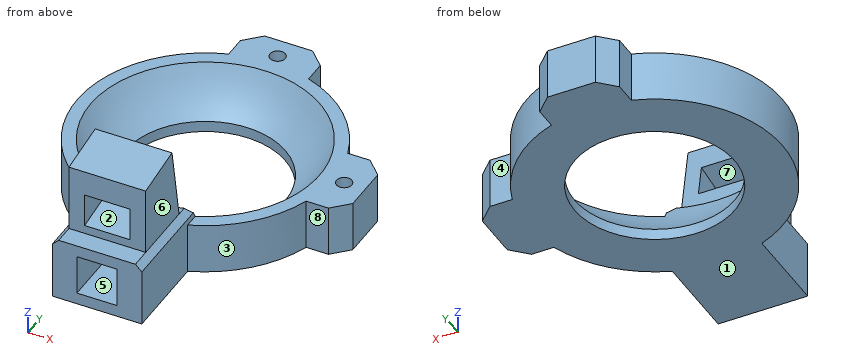
from build123d import *

# Parameters (mm, degrees)
SKETCH1_R            = 12.5
BOSS_EXTRUDE1_DEPTH  = 8
BOSS_EXTRUDE2_DEPTH  = 10
SKETCH4_W            = 6.3
SKETCH4_H            = 6.3
CUT_EXTRUDE1_DEPTH   = 12
BOSS_EXTRUDE4_DEPTH  = 6
SKETCH13_W           = 7.1
SKETCH13_H           = 5.2
CUT_EXTRUDE5_DEPTH   = 51.192153127
SKETCH22_W           = 12.489995996
SKETCH22_H           = 4
BOSS_EXTRUDE10_DEPTH = 8
SKETCH24_R           = 1.2
CUT_EXTRUDE8_DEPTH   = 6.5
CIRPATTERN1_COUNT    = 2
CIRPATTERN1_ANGLE    = 90
CHAMFER1_SIZE        = 2.5
CHAMFER2_SIZE        = 1


with BuildPart() as part:
    # Sketch1 → Boss-Extrude1 (new body)
    with BuildSketch(Plane.XY):
        with BuildLine():
            Line((-6.244997998, 21), (6.244997998, 21))
            Line((6.244997998, 21), (6.244997998, 19))
            ThreePointArc((6.244997998, 19), (14.142135624, 14.142135624), (19, 6.244997998))
            Line((19, 6.244997998), (21, 6.244997998))
            Line((21, 6.244997998), (21, -6.244997998))
            Line((21, -6.244997998), (19, -6.244997998))
            ThreePointArc((19, -6.244997998), (11.728172066, -16.200308021), (0, -20))
            ThreePointArc((0, -20), (-19.748417658, -3.16227766), (-6.244997998, 19))
            Line((-6.244997998, 19), (-6.244997998, 21))
        make_face()
        Circle(SKETCH1_R, mode=Mode.SUBTRACT)
    extrude(amount=BOSS_EXTRUDE1_DEPTH)

    # Sketch3 → Boss-Extrude2 (add)
    with BuildSketch(Plane.XY):
        Polygon((-7, -18.734993995), (-7, -32.5), (7, -32.5), (7, -18.734993995), (7, -15.234993995), (-7, -15.234993995), align=None)
    extrude(amount=BOSS_EXTRUDE2_DEPTH)

    # Sketch2 → Cut-Revolve2 (revolve, cut)
    with BuildSketch(Plane(origin=(0, 0, 0), x_dir=(1, 0, 0), z_dir=(0, 1, 0))):
        with BuildLine():
            Line((0, -38.5), (0, 2.5))
            ThreePointArc((0, 2.5), (-20.5, -18), (0, -38.5))
        make_face()
    revolve(axis=Axis((0, 0, 8), (0, 0, -1)), mode=Mode.SUBTRACT)

    # Sketch4 → Cut-Extrude1 (cut)
    with BuildSketch(Plane.XZ.offset(32.5)):
        with Locations((0, 5)):
            Rectangle(SKETCH4_W, SKETCH4_H)
    extrude(amount=-CUT_EXTRUDE1_DEPTH, mode=Mode.SUBTRACT)

    # Sketch11 → Boss-Extrude4 (add, symmetric)
    with BuildSketch(Plane(origin=(0, 0, 0), x_dir=(0, 0, -1), z_dir=(1, 0, 0))):
        Polygon((-10, -19.405629698), (-22, -21.521553466), (-20.609824642, -29.405629698), (-10, -29.405629698), align=None)
    extrude(amount=BOSS_EXTRUDE4_DEPTH, both=True)

    # Sketch13 → Cut-Extrude5 (cut, through all)
    with BuildSketch(Plane(origin=(0, -17.110377647, -3.017021229), x_dir=(1, 0, 0), z_dir=(0, 0.9848077530122074, 0.17364817766693455))):
        with Locations((0, -18.884652651)):
            Rectangle(SKETCH13_W, SKETCH13_H)
    extrude(amount=-CUT_EXTRUDE5_DEPTH, mode=Mode.SUBTRACT)

    # Sketch22 → Boss-Extrude10 (add)
    with BuildSketch(Plane.XY):
        with Locations((0, 23)):
            Rectangle(SKETCH22_W, SKETCH22_H)
    boss_extrude10 = extrude(amount=BOSS_EXTRUDE10_DEPTH)

    # Sketch24 → Cut-Extrude8 (cut)
    with BuildSketch(Plane.XY.offset(8)):
        with Locations((0, 21.7)):
            Circle(SKETCH24_R)
    cut_extrude8 = extrude(amount=-CUT_EXTRUDE8_DEPTH, mode=Mode.SUBTRACT)

    # CirPattern1: Boss-Extrude10, Cut-Extrude8 ×2 about axis
    cirpattern1_axis = Axis((0, 0, 0), (0, 0, -1))
    add([boss_extrude10.rotate(cirpattern1_axis, i * CIRPATTERN1_ANGLE / (CIRPATTERN1_COUNT - 1)) for i in range(1, CIRPATTERN1_COUNT)])
    add([cut_extrude8.rotate(cirpattern1_axis, i * CIRPATTERN1_ANGLE / (CIRPATTERN1_COUNT - 1)) for i in range(1, CIRPATTERN1_COUNT)], mode=Mode.SUBTRACT)

    # Chamfer1
    chamfer1_edges = [part.edges().sort_by_distance(p)[0] for p in [
        (-6.244997998, 25, 4),
        (6.244997998, 25, 4),
        (25, 6.244997998, 4),
        (25, -6.244997998, 4),
    ]]
    chamfer(chamfer1_edges, length=CHAMFER1_SIZE)

    # Chamfer2
    chamfer2_edges = [part.edges().sort_by_distance(p)[0] for p in [
        (7, -25.014274071, 10),
        (-7, -25.014274071, 10),
    ]]
    chamfer(chamfer2_edges, length=CHAMFER2_SIZE - 0.0001)  # a hair under: the kernel refuses the full size


solid = part.part
The model under review builds one solid part; all positions refer to its coordinate system, in mm. Face numbers are marked on the shaded views. A direction names the side the tool comes from. Give positions to 0.01 mm unless a question says otherwise; leave off trailing zeros. Loops run counter-clockwise (first coordinate to the right, second up) from the corner with the lowest first, then second, coordinate; pieces in that order, holes last. Notation, with made-up numbers: (0, 80) -> (24, 80) arc R16 ccw to (24, 101) -> close; hole circle Ø3 at (-19, 12). An arc over 180 degrees is marked (long way). Put each result on its own line as item: value. Start each with the question number.
1. Mouldability with a two-part tool opening along Z and no side actions: class the marked faces 1, 2 and 3 as released by +Z, released by -Z, zero draft, split by the parting line, or undercut.
2. We need section C-C on x = 0. State the section outline as (y, z) points.
3. We need section A-A on y = 0. State the section outline as (x, z) points, then the cut area to 3 significant figures.
4. We need section D-D on y = 21.7. State the section outline as (x, z) points (3 decimals), then the cut area to 3 significant figures.
5. Clearance check with flat-ended pins moving along their axes: P1, Ø1.9, axis at x = 21, y = -0.5, coming from the +Z side; P2, Ø2.5, axis at y = -26, z = 5, coming from the +X side; P3, Ø10, axis at x = 13.5, z = 19, coming from the +Y side; P4, Ø2, axis at y = -26, z = 14.5, coming from the -X side. State where each tip first meets the part, or that it passes through.
6. For the marked faces 4, 5, 6, 7 and 8, list the 3-axis set-ups (+Z, -Z, +X, -X, +Y, -Y) from which the entire face can be reached by the end or side of a thin tool; tool diameter is ignored.
7. We need section B-B on z = 15.25. State the section outline as (x, y) points.
8. Wall thickness on probe 1 along Y at (x, z) = (0, 6.25); probe 2 along X at (y, z) = (-25, 16.25); probe 3 along X at (y, z) = (-21.5, 6.75): over which ranges is each line inside the solid? List them lowest first.
Determined:
1. face 1: released by -Z
1. face 2: undercut
1. face 3: zero draft
2. outline: (-32.5, 0) -> (-12.5, 0) -> (-12.5, 1.75) arc R20.5 cw to (-18.87, 10) -> (-19.41, 10) -> (-19.94, 13.02) -> (-29.41, 11.35) -> (-29.41, 10) -> (-32.5, 10) -> (-32.5, 8.15) -> (-20.5, 8.15) -> (-20.5, 1.85) -> (-32.5, 1.85) -> close; (-29.41, 16.63) -> (-20.84, 18.14) -> (-21.52, 22) -> (-29.41, 20.61) -> close; (12.5, 0) -> (25, 0) -> (25, 8) -> (22.9, 8) -> (22.9, 1.5) -> (20.5, 1.5) -> (20.5, 8) -> (17.9, 8) arc R20.5 cw to (12.5, 1.75) -> close
3. outline: (-20, 0) -> (-12.5, 0) -> (-12.5, 1.75) arc R20.5 cw to (-17.9, 8) -> (-20, 8) -> close; (12.5, 0) -> (25, 0) -> (25, 8) -> (22.9, 8) -> (22.9, 1.5) -> (20.5, 1.5) -> (20.5, 8) -> (17.9, 8) arc R20.5 cw to (12.5, 1.75) -> close
3. area: 106 mm^2
4. outline: (-6.245, 0) -> (6.245, 0) -> (6.245, 8) -> (1.2, 8) -> (1.2, 1.5) -> (-1.2, 1.5) -> (-1.2, 8) -> (-6.245, 8) -> close
4. area: 84.3 mm^2
5. P1: z = 8
5. P2: x = 7
5. P3: through
5. P4: x = -6
6. face 4: +Z, -Z, +X, +Y
6. face 5: -Y
6. face 6: +Z, +X, +Y, -Y
6. face 7: +Y
6. face 8: +Z, -Z, +X, -Y
7. outline: (-6, -29.41) -> (-3.55, -29.41) -> (-3.55, -20.33) -> (-6, -20.33) -> close; (3.55, -29.41) -> (6, -29.41) -> (6, -20.33) -> (3.55, -20.33) -> close
8. probe 1: -20.5 to -16.8, 16.8 to 20.5, 22.9 to 25
8. probe 2: -6 to -3.55, 3.55 to 6
8. probe 3: -7 to -3.15, 3.15 to 7
